from build123d import *

# Parameters (mm, degrees)
F0_W     = 25.4
F0_H     = 1270
F1_DEPTH = 25.4
F2_W     = 1625.6
F2_H     = 1320.8
F3_DEPTH = 6.35
F4_R     = 9.525
F5_DEPTH = 1320.8
F6_W     = 50.8
F6_H     = 1270
F7_DEPTH = 1625.601


with BuildPart() as f1:
    # F0 (on Front) → F1 (new body)
    with BuildSketch(Plane.XZ):
        with Locations((787.4, 300.803003)):
            Rectangle(F0_W, F0_H)
        Polygon((1600.2, 961.203003), (-25.4, 961.203003), (-25.4, 935.803003), (0, 935.803003), (774.7, 935.803003), (800.1, 935.803003), (1574.8, 935.803003), (1600.2, 935.803003), align=None)
        with Locations((-12.7, 300.803003)):
            Rectangle(F0_W, F0_H)
        Polygon((0, -334.196997), (-25.4, -334.196997), (-25.4, -359.596997), (1600.2, -359.596997), (1600.2, -334.196997), (1574.8, -334.196997), (800.1, -334.196997), (774.7, -334.196997), align=None)
        with Locations((1587.5, 300.803003)):
            Rectangle(F0_W, F0_H)
    extrude(amount=F1_DEPTH)

    # F2 (on face) → F3 (join)
    with BuildSketch(Plane.XZ.offset(25.4)):
        with Locations((787.4, 300.803003)):
            Rectangle(F2_W, F2_H)
    extrude(amount=F3_DEPTH)

    # F4 (on face) → F5 (join)
    with BuildSketch(Plane(origin=(0, 0, -359.596997), x_dir=(1, 0, 0), z_dir=(0, 0, -1))):
        with BuildLine():
            Line((177.8, 0), (127, 0))
            Line((127, 0), (127, -6.35))
            Line((127, -6.35), (127, -25.4))
            ThreePointArc((127, -25.4), (134.439488, -43.360512), (152.4, -50.8))
            ThreePointArc((152.4, -50.8), (170.360512, -43.360512), (177.8, -25.4))
            Line((177.8, -25.4), (177.8, -6.35))
            Line((177.8, -6.35), (177.8, 0))
        make_face()
        with Locations((152.4, -25.4)):
            Circle(F4_R, mode=Mode.SUBTRACT)
        with BuildLine():
            Line((127, -6.35), (127, 0))
            Line((127, 0), (101.6, 0))
            ThreePointArc((101.6, 0), (103.459872, -4.490128), (107.95, -6.35))
            Line((107.95, -6.35), (127, -6.35))
        make_face()
        with BuildLine():
            Line((203.2, 0), (177.8, 0))
            Line((177.8, 0), (177.8, -6.35))
            Line((177.8, -6.35), (196.85, -6.35))
            ThreePointArc((196.85, -6.35), (201.340128, -4.490128), (203.2, 0))
        make_face()
        with BuildLine():
            Line((1447.8, -6.35), (1447.8, 0))
            Line((1447.8, 0), (1397, 0))
            Line((1397, 0), (1397, -6.35))
            Line((1397, -6.35), (1397, -25.4))
            ThreePointArc((1397, -25.4), (1404.439488, -43.360512), (1422.4, -50.8))
            ThreePointArc((1422.4, -50.8), (1440.360512, -43.360512), (1447.8, -25.4))
            Line((1447.8, -25.4), (1447.8, -6.35))
        make_face()
        with Locations((1422.4, -25.4)):
            Circle(F4_R, mode=Mode.SUBTRACT)
        with BuildLine():
            Line((1473.2, 0), (1447.8, 0))
            Line((1447.8, 0), (1447.8, -6.35))
            Line((1447.8, -6.35), (1466.85, -6.35))
            ThreePointArc((1466.85, -6.35), (1471.340128, -4.490128), (1473.2, 0))
        make_face()
        with BuildLine():
            Line((1397, -6.35), (1397, 0))
            Line((1397, 0), (1371.6, 0))
            ThreePointArc((1371.6, 0), (1373.459872, -4.490128), (1377.95, -6.35))
            Line((1377.95, -6.35), (1397, -6.35))
        make_face()
    extrude(amount=-F5_DEPTH)

    # F6 (on face) → F7 (cut, through all)
    with BuildSketch(Plane.YZ.offset(1600.2)):
        with Locations((25.4, 300.803003)):
            Rectangle(F6_W, F6_H)
    extrude(amount=-F7_DEPTH, mode=Mode.SUBTRACT)


solid = f1.part
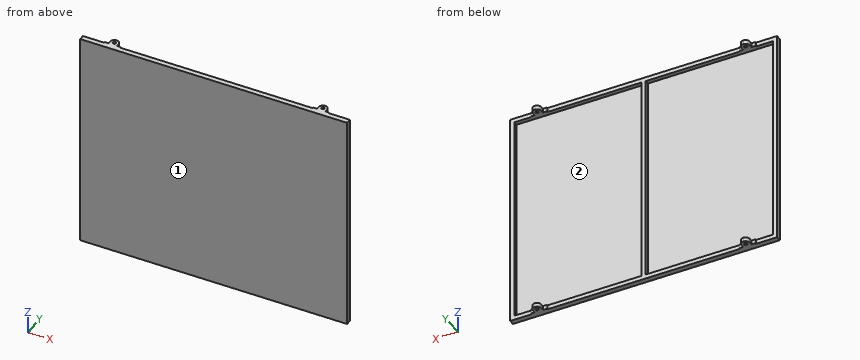
Read the model definition and answer for the solid it produces. Units are mm, in the model's axes. Face numbers are marked on the shaded views. Round coordinates to 2 decimals unless told otherwise and drop trailing zeros. Loops run counter-clockwise (first coordinate to the right, second up) from the corner with the lowest first, then second, coordinate; pieces in that order, holes last.
Q1. Section B-B on z = 786 is taken. Write down the section's boundary in (x, y).
Q2. Each of these flat-tipped pins is pushed along its axis until it touches: pin 1 (25 mm diameter, centred on x = 1422.4, y = 25.4, fed in from -Z); pin 2 (1.5 mm diameter, centred on x = 1052.5, z = 171.5, fed in from +Y); pin 3 (5.5 mm diameter, centred on y = 16, z = -344.5, fed in from -X); pin 4 (21 mm diameter, centred on x = 1454.5, z = -348, fed in from +Y). Where does it stop, or does it pass through?
Q3. Determine the mould class of the marked faces 1 and 2 for opening direction X: released by +X, released by -X, zero draft, split by the parting line, or undercut.
Q4. Section A-A on x = 1138.5 is taken. Write down the section's boundary in (y, z).
Q5. Consider probe 1 along X at (y, z) = (25.4, 954) (3 decimals); probe 2 along X at (y, z) = (-4, 125); probe 3 along Y at (x, z) = (1422.4, -352.75) (3 decimals). Determine where each line is inside the solid, lowest interval first.
Output:
1. outline: (-25.4, -31.75) - (1600.2, -31.75) - (1600.2, 0) - (1574.8, 0) - (1574.8, -25.4) - (800.1, -25.4) - (800.1, 0) - (774.7, 0) - (774.7, -25.4) - (0, -25.4) - (0, 0) - (-25.4, 0) - close
2. pin 1: stops at z = -359.6
2. pin 2: stops at y = -25.4
2. pin 3: stops at x = 127
2. pin 4: stops at y = 38.76
3. face 1: zero draft
3. face 2: undercut
4. outline: (-31.75, -359.6) - (0, -359.6) - (0, -334.2) - (-25.4, -334.2) - (-25.4, 935.8) - (0, 935.8) - (0, 961.2) - (-31.75, 961.2) - close
5. probe 1: x = 127 to 142.875, 161.925 to 177.8, 1397 to 1412.875, 1431.925 to 1447.8
5. probe 2: x = -25.4 to 0, 774.7 to 800.1, 1574.8 to 1600.2
5. probe 3: y = -31.75 to 15.875, 34.925 to 50.8
